Autodesk Inventor part; units mm, degrees
ref_plane "YZ Plane" through (0, 0, 0) normal (1, 0, 0) x (0, 1, 0)
ref_plane "XZ Plane" through (0, 0, 0) normal (0, 1, 0) x (-1, 0, 0)
ref_plane "XY Plane" through (0, 0, 0) normal (0, 0, 1) x (1, 0, 0)
sketch "Sketch1" plane through (0, 0, 0) normal (0, 1, 0) x (-1, 0, 0)
  circle A0 centre (0, 0) radius 40
  dimension "d0" = 80
extrude "Extrusion1" add sketch "Sketch1" along normal blind 20
sketch "Sketch2" plane through (0, 20, 0) normal (0, 1, 0) x (1, 0, 0)
  circle A0 centre (0, 0) radius 40
  line L0 (-56, 0) -> (56, 0)
  line L1 (0, 56) -> (0, -56)
  circle A1 centre (-20, -20) radius 5
  dimension "d3" = 10
  dimension "d4" = 20
  dimension "d5" = 20
extrude "Extrusion2" cut sketch "Sketch2" against normal through all contours A1
sketch "Sketch3" plane through (0, 20, 0) normal (0, 1, 0) x (1, 0, 0)
  circle A0 centre (0, 0) radius 5
  dimension "d8" = 10
extrude "Extrusion3" cut sketch "Sketch3" against normal through all
equation "\"d6\" = d3"
equation "\"d9\" = d3"
properties part number "flywheel"
Geometry check sheet. Reference: the model listing, model coordinates, mm. Round coordinates to 2 decimals unless told otherwise and drop trailing zeros. Order: outer loops, then holes, each group sorted by start corner. A loop starts at its lowest first (then second) coordinate and runs counter-clockwise, first axis right, second up. Notation, with made-up numbers: M 81,-12 L 110,-12 A11 cw 110,-2 Z; hole C -12.75,73.5 d5. An arc over 180 degrees is marked long. Answer in a Markdown table with one row per item. Add a question column.
Item 1: Sectioned sample at A-A, the plane z = 0. Enter the section's corners in (x, y), plus the area to 3 significant figures.
Item 2: Sectioned sample at B-B, the plane x = 0. Enter the section's corners in (y, z), plus the area to 3 significant figures.
Item 3: Material ranges on L1, parallel to Z at x = 0, y = 16; L2, parallel to X at y = 16, z = 21; L3, parallel to X at y = 13, z = 20, recorded low to high. Write a range as [from, to].
Item 4: Draft check along Z on faces 1 (the face through (-21.08, 10.14, 24.88)), 2 (the face through (1, 0, -8)), 3 (the face through (8.67, 9.86, 39.05)). Enter one of: released by +Z, released by -Z, zero draft, split by the parting line, or undercut.
Item 5: Sectioned sample at D-D, the plane x = -9. Enter the section's corners in (y, z), plus the area to 3 significant figures.
Item 6: Sectioned sample at C-C, the plane y = 17. Enter the section's corners in (x, z), plus the area to 3 significant figures.
Item 7: Depth check by flat-ended pin: pin 1 Ø1.5 at (y, z) = (16, 2.5) entering from -X; pin 2 Ø10 at (x, y) = (-14.5, 2.5) entering from +Z; pin 3 Ø6 at (x, y) = (26.5, 10) entering from +Z. Enter the tip coordinate at first touch or a pass-through.
Filled in:
| question | item | result |
|---|---|---|
| 1 | outline | M -40,0 L -5,0 L -5,20 L -40,20 Z; M 5,0 L 40,0 L 40,20 L 5,20 Z |
| 1 | area | 1,400 mm² |
| 2 | outline | M 0,-40 L 20,-40 L 20,-5 L 0,-5 Z; M 0,5 L 20,5 L 20,40 L 0,40 Z |
| 2 | area | 1,400 mm² |
| 3 | L1 | z = [-40, -5], [5, 40] |
| 3 | L2 | x = [-34.04, -24.9], [-15.1, 34.04] |
| 3 | L3 | x = [-34.64, -25], [-15, 34.64] |
| 4 | face 1 | undercut |
| 4 | face 2 | zero draft |
| 4 | face 3 | split by the parting line |
| 5 | outline | M 0,-38.97 L 20,-38.97 L 20,38.97 L 0,38.97 Z |
| 5 | area | 1,560 mm² |
| 6 | outline | C 0,0 d80; hole C -20,20 d10; hole C 0,0 d10 |
| 6 | area | 4,870 mm² |
| 7 | pin 1 | stops at x = -39.96 |
| 7 | pin 2 | stops at z = 38.86 |
| 7 | pin 3 | stops at z = 32.37 |
